Source: CAD feature listing. Evaluate the final solid. Frame: model axes, mm. A direction names the side the tool comes from. Coordinates: 2 decimals unless noted, no trailing zeros. Loops run counter-clockwise (first coordinate to the right, second up) from the corner with the lowest first, then second, coordinate; pieces in that order, holes last.
```python
from build123d import *

# Parameters (mm, degrees)
F0_W      = 140.1769816875
F0_H      = 53.487598896
F13_DEPTH = 131.8847630173
F1_DEPTH  = 69.7684045881
F2_DEPTH  = 56.6403288394
F14_DEPTH = 101.1081095785
F15_DEPTH = 68.6891395599
F4_R      = 17.78
F5_R      = 15.24
F6_DEPTH  = 28.8777854294
F10_DEPTH = 25.4
F12_DEPTH = 25.4


with BuildPart() as f13:
    # F0 (on Top) → F13 (new body)
    with BuildSketch(Plane.XY):
        Rectangle(F0_W, F0_H)
    extrude(amount=F13_DEPTH)

    # F1 (add): a face of the model
    f1_faces = [f13.faces().sort_by_distance(p)[0] for p in [
        (-70.0884908438, 0, 65.9423815086),
    ]]
    extrude(f1_faces, amount=F1_DEPTH)

    # F2 (add): a face of the model
    f2_faces = [f13.faces().sort_by_distance(p)[0] for p in [
        (70.0884908438, 0, 65.9423815086),
    ]]
    extrude(f2_faces, amount=F2_DEPTH)

    # F3 (on face) → F14 (cut)
    with BuildSketch(Plane.XZ.offset(26.743799448)):
        with BuildLine():
            Line((-83.9332714677, 0), (81.0228064656, 0))
            ThreePointArc((81.0228064656, 0), (-1.455232501, 108.6675575463), (-83.9332714677, 0))
        make_face()
    extrude(amount=-F14_DEPTH, mode=Mode.SUBTRACT)

    # F15 (add): a face of the model
    f15_faces = [f13.faces().sort_by_distance(p)[0] for p in [
        (-111.8950834498, -26.743799448, 2.9742483793),
    ]]
    extrude(f15_faces, amount=F15_DEPTH)

    # F4
    f4_edges = [f13.edges().sort_by_distance(p)[0] for p in [
        (-1.455233, 26.743799, 108.667558),
        (-1.455233, -95.432939, 108.667558),
    ]]
    fillet(f4_edges, radius=F4_R)

    # F5
    f5_edges = [f13.edges().sort_by_distance(p)[0] for p in [
        (126.72882, -95.432939, 65.942382),
        (126.72882, 26.743799, 65.942382),
        (-139.856895, -95.432939, 65.942382),
        (-139.856895, 26.743799, 65.942382),
    ]]
    fillet(f5_edges, radius=F5_R)

    # F16 (on face) → F6 (join)
    with BuildSketch(Plane.XY.offset(131.8847630173)):
        with BuildLine():
            ThreePointArc((111.4888196832, -95.4329390079), (122.2651270285, -90.9692463532), (126.7288196832, -80.1929390079))
            Line((126.7288196832, -80.1929390079), (-139.8568954319, -80.1929390079))
            ThreePointArc((-139.8568954319, -80.1929390079), (-135.3932027772, -90.9692463532), (-124.6168954319, -95.4329390079))
            Line((-124.6168954319, -95.4329390079), (111.4888196832, -95.4329390079))
        make_face()
        with BuildLine():
            Line((-139.8568954319, 11.503799448), (126.7288196832, 11.503799448))
            ThreePointArc((126.7288196832, 11.503799448), (122.2651270285, 22.2801067933), (111.4888196832, 26.743799448))
            Line((111.4888196832, 26.743799448), (-124.6168954319, 26.743799448))
            ThreePointArc((-124.6168954319, 26.743799448), (-135.3932027772, 22.2801067933), (-139.8568954319, 11.503799448))
        make_face()
    extrude(amount=F6_DEPTH)

    # F9 (on face) → F10 (cut)
    with BuildSketch(Plane.XZ.offset(95.4329390079)):
        with BuildLine():
            Line((-39.3435060978, 135.2504938841), (-0.6112582661, 135.2504938841))
            ThreePointArc((-0.6112582661, 135.2504938841), (-61.0826207458, 147.45574623), (-121.5539832255, 135.2504938841))
            Line((-121.5539832255, 135.2504938841), (-39.3435060978, 135.2504938841))
        make_face()
    extrude(amount=-F10_DEPTH, mode=Mode.SUBTRACT)

    # F11 (on face) → F12 (cut)
    with BuildSketch(Plane.XZ.offset(95.4329390079)):
        with BuildLine():
            Line((9.9441353232, 135.2504938841), (111.4393852922, 135.2504938841))
            ThreePointArc((111.4393852922, 135.2504938841), (56.4007480003, 150.371931024), (1.3621107084, 135.2504938841))
            Line((1.3621107084, 135.2504938841), (9.9441353232, 135.2504938841))
        make_face()
    extrude(amount=-F12_DEPTH, mode=Mode.SUBTRACT)


solid = f13.part
```
Q1. Section query A-A on y = -60. Return the cut outline in (x, z).
Q2. First-contact query: pin 1 Ø1 at (x, y) = (48.5, -49) entering from -Z; pin 2 Ø5 at (x, y) = (67, -49.5) entering from -Z; pin 3 Ø5 at (x, y) = (-13, 0) entering from -Z. Flat tips, straight axial feed; report the tip coordinate or a pass-through.
Q3. Draft query along Y for faces 1 (the flat face through (-8, 11.504, 146)), 2 (the cylindrical face through (0.75, -33.74, 108.64)), 3 (the flat face through (-34, 26.744, 133)). Return one class per face: released by +Y, released by -Y, zero draft, split by the parting line, or undercut.
Q4. Section query B-B on z = 144. Return the cut outline in (x, y).
Q5. Material intervals for line 1 along X through (y, z) = (-51.5, 23); line 2 along X through (y, z) = (4, 20.5); line 3 along Z through (x, y) = (-123.5, -10.5), sorted ascending.
Q6. Reachability of faces 4 (the flat face through (-5, -80.193, 149)), 5 (the flat face through (56, -88, 135.25)), 6 (the flat face through (104, -33, 0)) from +Z, -Z, +X, -X, +Y, -Y: full face, straight path, thin tool, end or side. Return the list, or none.
Resolved:
1. outline: (-139.86, 0) - (-83.93, 0) arc R85.63 cw (long way) to (81.02, 0) - (126.73, 0) - (126.73, 131.88) - (-139.86, 131.88) - close
2. pin 1: stops at z = 92.22
2. pin 2: stops at z = 70.98
2. pin 3: stops at z = 107.51
3. face 1: undercut
3. face 2: zero draft
3. face 3: released by +Y
4. outline: (-139.86, -80.19) arc R15.24 ccw to (-124.62, -95.43) - (-93.73, -95.43) - (-93.73, -80.19) - close; (-139.86, 11.5) - (126.73, 11.5) arc R15.24 ccw to (111.49, 26.74) - (-124.62, 26.74) arc R15.24 ccw to start; (-28.44, -95.43) - (19.9, -95.43) - (19.9, -80.19) - (-28.44, -80.19) - close; (92.9, -95.43) - (111.49, -95.43) arc R15.24 ccw to (126.73, -80.19) - (92.9, -80.19) - close
5. line 1: x = -139.86 to -87.09, 84.18 to 126.73
5. line 2: x = -139.86 to -87.05, 84.14 to 126.73
5. line 3: z = 0 to 131.88
6. face 4: +Z, +X, -X
6. face 5: -Y
6. face 6: -Z, +X, -X, +Y, -Y
